```python
from build123d import *

# Parameters (mm, degrees)
BOSS_EXTRUDE1_DEPTH = 6
SKETCH2_R           = 422.5
CUT_EXTRUDE1_DEPTH  = 6
SKETCH3_R           = 4.5
CUT_EXTRUDE2_DEPTH  = 6
CIRPATTERN1_COUNT   = 16
SKETCH4_R           = 3
CUT_EXTRUDE3_DEPTH  = 10
SKETCH5_R           = 7.5
CUT_EXTRUDE4_DEPTH  = 10
FILLET1_R           = 6


with BuildPart() as part:
    # Sketch1 → Boss-Extrude1 (new body)
    with BuildSketch(Plane(origin=(0, 0, 0), x_dir=(1, 0, 0), z_dir=(0, 1, 0))):
        Polygon((315.066450454, 496.5), (497.5, 314.066450454), (497.5, -315.066450454), (315.066450454, -497.5), (-314.066450454, -497.5), (-496.5, -315.066450454), (-496.5, 314.066450454), (-314.066450454, 496.5), align=None)
    extrude(amount=BOSS_EXTRUDE1_DEPTH)

    # Sketch2 → Cut-Extrude1 (cut)
    with BuildSketch(Plane(origin=(0, 6, 0), x_dir=(1, 0, 0), z_dir=(0, 1, 0))):
        with Locations(Location((0, 0, 0), (0, 0, 270))):
            Circle(SKETCH2_R)
    extrude(amount=-CUT_EXTRUDE1_DEPTH, mode=Mode.SUBTRACT)

    # Sketch3 → Cut-Extrude2 (cut)
    with BuildSketch(Plane(origin=(0, 6, 0), x_dir=(1, 0, 0), z_dir=(0, 1, 0))):
        with Locations(Location((0, 442.5, 0), (0, 0, 270))):
            Circle(SKETCH3_R)
    cut_extrude2 = extrude(amount=-CUT_EXTRUDE2_DEPTH, mode=Mode.SUBTRACT)

    # CirPattern1: Cut-Extrude2 ×16 about axis
    cirpattern1_axis = Axis((0, 0, 0), (0, 1, 0))
    for i in range(1, CIRPATTERN1_COUNT):
        add(cut_extrude2.rotate(cirpattern1_axis, i * 360 / CIRPATTERN1_COUNT), mode=Mode.SUBTRACT)

    # Sketch4 → Cut-Extrude3 (cut)
    with BuildSketch(Plane(origin=(0, 6, 0), x_dir=(1, 0, 0), z_dir=(0, 1, 0))):
        with Locations(Location((445.5, 262.066450454, 0), (0, 0, 270))):
            Circle(SKETCH4_R)
    extrude(amount=-CUT_EXTRUDE3_DEPTH, mode=Mode.SUBTRACT)

    # Sketch5 → Cut-Extrude4 (cut)
    with BuildSketch(Plane(origin=(0, 6, 0), x_dir=(1, 0, 0), z_dir=(0, 1, 0))):
        with Locations(Location((-461.5, 244.066450454, 0), (0, 0, 270))):
            Circle(SKETCH5_R)
        with Locations(Location((462.5, -245.066450454, 0), (0, 0, 270))):
            Circle(SKETCH5_R)
    extrude(amount=-CUT_EXTRUDE4_DEPTH, mode=Mode.SUBTRACT)

    # Fillet1
    fillet1_edges = [part.edges().sort_by_distance(p)[0] for p in [
        (315.066450454, 3, -496.5),
        (497.5, 3, -314.066450454),
        (497.5, 3, 315.066450454),
        (315.066450454, 3, 497.5),
        (-314.066450454, 3, 497.5),
        (-496.5, 3, 315.066450454),
        (-496.5, 3, -314.066450454),
        (-314.066450454, 3, -496.5),
    ]]
    fillet(fillet1_edges, radius=FILLET1_R)


solid = part.part
```
Check sheet for the modelled part. Datum: model origin and axes. Units: mm. Coordinates: 2 decimals unless noted, no trailing zeros. Order: outer loops, then holes, each group sorted by start corner. A loop starts at its lowest first (then second) coordinate and runs counter-clockwise, first axis right, second up. Notation, with made-up numbers: M 74,16.5 L 78,16.5 A34 cw 78,48.5 Z; hole C 4.5,85.5 d4. An arc over 180 degrees is marked long. Write each question's results on one line, items separated by ' | '. Start each with the question number.
1. Cross-section at B-B on x = 329. Record the cut outline in (y, z), and give its area (3 significant figures).
2. Material ranges on probe 1 along Z at (x, y) = (315, 5.25); probe 2 along X at (y, z) = (2.5, -4); probe 3 along Z at (x, y) = (123, 3.1), recorded low to high.
3. Go/stop test with a flat-tipped pin: P1, Ø3.5, axis at x = 445.5, z = -262.07, coming from the -Y side. Record where the tip stops, or that it passes through.
4. Cross-section at C-C on y = 1. State how many separate pieces and enclosed holes the cut face has, and give its area (3 significant figures).
5. Cross-section at A-A on z = 376. Record the cut outline in (x, y), and give its area (3 significant figures).
6. Mould release check, pull along X, two halves, no side actions. Record for faces 1 (the face through (-412.453, 3.042, -91.59)), 2 (the face through (407.536, 2.958, 405.031)), 3 (the face through (-404.031, 2.958, 407.536)), 4 (the face through (449, 6, -6)): +X half, -X half, draft (parallel to the pull), parting line (faces both ways), or undercut.
Checks:
1) outline: M 0,-482.57 L 6,-482.57 L 6,-265.08 L 0,-265.08 Z; M 0,265.08 L 6,265.08 L 6,483.57 L 0,483.57 Z | area: 2,620 mm²
2) probe 1: z = -495.99 to -316.87, -308.92 to -281.57, 281.57 to 308.92, 316.87 to 496.99 | probe 2: x = -496.5 to -444.56, -440.44 to -422.48, 422.48 to 440.44, 444.56 to 497.5 | probe 3: z = -496.5 to -404.2, 404.2 to 497.5
3) P1: passes through
4) separate pieces: 1 | enclosed holes: 20 | area: 359,000 mm²
5) outline: M -435.57,0 L -192.69,0 L -192.69,6 L -435.57,6 Z; M 192.69,0 L 436.57,0 L 436.57,6 L 192.69,6 Z | area: 2,920 mm²
6) face 1: undercut | face 2: +X half | face 3: -X half | face 4: draft
